Here's how the part is built. I have some questions about the finished solid (model axes, mm). A direction names the side the tool comes from. Give positions to 0.01 mm unless a question says otherwise; leave off trailing zeros. Loops run counter-clockwise (first coordinate to the right, second up) from the corner with the lowest first, then second, coordinate; pieces in that order, holes last. Notation, with made-up numbers: (31, 29) - (54, 29) arc R30 cw to (54, 60) - close; hole circle Ø6 at (41, 13). An arc over 180 degrees is marked (long way). Use a Markdown table: item, result.
from build123d import *

# Parameters (mm, degrees)
PAD_DEPTH       = 6
POCKET_DEPTH    = 3
SKETCH002_W     = 18.4
SKETCH002_H     = 20.85
POCKET001_DEPTH = 3
SKETCH003_W     = 8.55
SKETCH003_H     = 1.65
POCKET002_DEPTH = 3
PAD001_DEPTH    = 3


with BuildPart() as part:
    # Sketch → Pad (new body)
    with BuildSketch(Plane.XY):
        with BuildLine():
            ThreePointArc((-75, 28.5), (-103.5, 0), (-75, -28.5))
            Line((-75, -28.5), (75, -28.5))
            ThreePointArc((75, -28.5), (103.5, 0), (75, 28.5))
            Line((-75, 28.5), (75, 28.5))
        make_face()
    extrude(amount=PAD_DEPTH)

    # Sketch001 (on Face6 of Pad) → Pocket (cut)
    with BuildSketch(Plane.XY.offset(6)):
        with BuildLine():
            ThreePointArc((-62.5, 6), (-68.5, 0), (-62.5, -6))
            Line((-62.5, -6), (62.5, -6))
            ThreePointArc((62.5, -6), (68.5, 0), (62.5, 6))
            Line((-62.5, 6), (62.5, 6))
        make_face()
    extrude(amount=-POCKET_DEPTH, mode=Mode.SUBTRACT)

    # Sketch002 (on Face5 of Pocket) → Pocket001 (cut)
    with BuildSketch(Plane.XY.offset(6)):
        with Locations((0, -16.425)):
            Rectangle(SKETCH002_W, SKETCH002_H)
    extrude(amount=-POCKET001_DEPTH, mode=Mode.SUBTRACT)

    # Sketch003 (on Face5 of Pocket001) → Pocket002 (cut)
    with BuildSketch(Plane.XY.offset(6)):
        with Locations((0, -27.675)):
            Rectangle(SKETCH003_W, SKETCH003_H)
    extrude(amount=-POCKET002_DEPTH, mode=Mode.SUBTRACT)

    # Sketch004 (on Face5 of Pocket002) → Pad001 (join)
    with BuildSketch(Plane.XY.offset(6)):
        with BuildLine():
            ThreePointArc((-75, 28.5), (-103.5, 0), (-75, -28.5))
            Line((-75, -28.5), (75, -28.5))
            ThreePointArc((75, -28.5), (103.5, 0), (75, 28.5))
            Line((-75, 28.5), (75, 28.5))
        make_face()
        with BuildLine():
            ThreePointArc((-62.5, 6), (-68.5, 0), (-62.5, -6))
            Line((-62.5, -6), (62.5, -6))
            ThreePointArc((62.5, -6), (68.5, 0), (62.5, 6))
            Line((-62.5, 6), (62.5, 6))
        make_face(mode=Mode.SUBTRACT)
    extrude(amount=PAD001_DEPTH)


solid = part.part
(1) Suppose I cut it at A-A on y = -13. Write out the boundary of the cut face in (x, z), plus the area to 3 significant figures.
A:
| item | result |
|---|---|
| outline | (-100.36, 0) - (100.36, 0) - (100.36, 9) - (-100.36, 9) - close; hole (-9.2, 3) - (9.2, 3) - (9.2, 6) - (-9.2, 6) - close |
| area | 1,750 mm2 |
(2) Suppose I cut it at D-D on y = -24. Write out the boundary of the cut face in (x, z), plus the area to 3 significant figures.
A:
| item | result |
|---|---|
| outline | (-90.37, 0) - (90.37, 0) - (90.37, 9) - (-90.37, 9) - close; hole (-9.2, 3) - (9.2, 3) - (9.2, 6) - (-9.2, 6) - close |
| area | 1,570 mm2 |
(3) We'd pull the mould along Z, two halves only. Please class faces 1 (the face through (-1, 7, 9)), 2 (the face through (-1, 0, 0)), 3 (the face through (-1, -3, 3)): pulls with the +Z half, pulls with the -Z half, needs draft (parallel to the pull), parting line crosses it, or undercut.
A:
| item | result |
|---|---|
| face 1 | pulls with the +Z half |
| face 2 | pulls with the -Z half |
| face 3 | undercut |
(4) Suppose I cut it at C-C on y = 0. Write out the boundary of the cut face in (x, z).
A:
| item | result |
|---|---|
| outline | (-103.5, 0) - (103.5, 0) - (103.5, 9) - (68.5, 9) - (68.5, 3) - (-68.5, 3) - (-68.5, 9) - (-103.5, 9) - close |
(5) If I drill on line 1 (Y direction, x = 21, z = 8.5); line 2 (Y direction, x = -6, z = 5.5); line 3 (X direction, y = 4.5, z = 4.75), over which ranges is the centre line in solid material (lowest first)?
A:
| item | result |
|---|---|
| line 1 | -28.5 to -6, 6 to 28.5 |
| line 2 | -28.5 to -26.85, 6 to 28.5 |
| line 3 | -103.14 to -66.47, 66.47 to 103.14 |
(6) Suppose I cut it at B-B on x = -23.5. Write out the boundary of the cut face in (y, z), plus the area to 3 significant figures.
A:
| item | result |
|---|---|
| outline | (-28.5, 0) - (28.5, 0) - (28.5, 9) - (6, 9) - (6, 3) - (-6, 3) - (-6, 9) - (-28.5, 9) - close |
| area | 441 mm2 |
(7) Will these pins go through, and if not, where does the flat tip stop? pin 1 (1 mm diameter, centred on x = -9, y = 2, fed in from +Z); pin 2 (2.5 mm diameter, centred on y = -19, z = 4, fed in from -X); pin 3 (1.5 mm diameter, centred on y = -16, z = 4.5, fed in from +X).
A:
| item | result |
|---|---|
| pin 1 | z = 3 |
| pin 2 | x = -97.3 |
| pin 3 | x = 99.08 |
(8) On a 3-axis mill with a long thin cutter (end or side, diameter ignored), from which of +Z, -Z, +X, -X, +Y, -Y can I reach the whole of each face in a straight line? I mean faces 4 (the face through (-1, -28.5, 6.4)), 5 (the face through (0, -17, 6)), 6 (the face through (-68.5, 0.1, 6)). Say none if no direction works.
A:
| item | result |
|---|---|
| face 4 | +Z, -Z, +X, -X, -Y |
| face 5 | none |
| face 6 | +Z |
